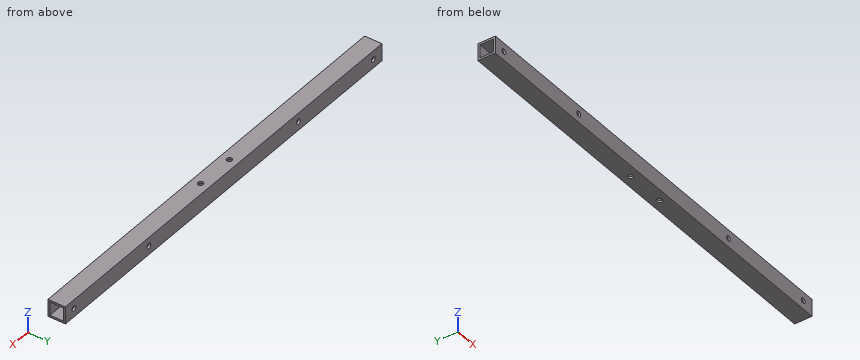
from build123d import *

# Parameters (mm, degrees)
SKETCH1_W           = 650
SKETCH1_H           = 26
BOSS_EXTRUDE1_DEPTH = 26
SHELL1_T            = -3
SKETCH2_R           = 4
CUT_EXTRUDE1_DEPTH  = 26
SKETCH3_R           = 4
CUT_EXTRUDE2_DEPTH  = 27


with BuildPart() as part:
    # Sketch1 → Boss-Extrude1 (new body)
    with BuildSketch(Plane(origin=(0, 0, 0), x_dir=(1, 0, 0), z_dir=(0, 1, 0))):
        Rectangle(SKETCH1_W, SKETCH1_H)
    extrude(amount=BOSS_EXTRUDE1_DEPTH)

    # Shell1
    shell1_openings = [part.faces().sort_by_distance(p)[0] for p in [
        (-325, 13, 0),
        (325, 13, 0),
    ]]
    offset(amount=SHELL1_T, openings=shell1_openings, kind=Kind.INTERSECTION)

    # Sketch2 → Cut-Extrude1 (cut)
    with BuildSketch(Plane(origin=(0, 26, 0), x_dir=(1, 0, 0), z_dir=(0, 1, 0))):
        with Locations((307.5, 0)):
            Circle(SKETCH2_R)
        with Locations((-307.5, 0)):
            Circle(SKETCH2_R)
        with Locations((153.75, 0)):
            Circle(SKETCH2_R)
        with Locations((-153.75, 0)):
            Circle(SKETCH2_R)
    extrude(amount=-CUT_EXTRUDE1_DEPTH, mode=Mode.SUBTRACT)

    # Sketch3 → Cut-Extrude2 (cut, through all)
    with BuildSketch(Plane.XY.offset(13)):
        with Locations((-29.5, 13)):
            Circle(SKETCH3_R)
        with Locations((29.5, 13)):
            Circle(SKETCH3_R)
    extrude(amount=-CUT_EXTRUDE2_DEPTH, mode=Mode.SUBTRACT)


solid = part.part
Geometry check sheet. Reference: the model listing, model coordinates, mm. Round coordinates to 2 decimals unless told otherwise and drop trailing zeros. Order: outer loops, then holes, each group sorted by start corner. A loop starts at its lowest first (then second) coordinate and runs counter-clockwise, first axis right, second up. Notation, with made-up numbers: M -27,41.5 L 18,41.5 A14 cw 18,53.5 Z; hole C -33,64 d8. An arc over 180 degrees is marked long. Write each question's results on one line, items separated by ' | '. Start each with the question number.
1. Material ranges on L1, parallel to X at y = 1.4, z = 0; L2, parallel to Y at x = 273.5, z = -7.5; L3, parallel to Z at x = -160.5, y = 10.25, recorded low to high. Write a range as from..to.
2. Go/stop test with flat-tipped pins: P1, Ø13, axis at x = -153.75, z = 0, coming from the -Y side; P2, Ø6.5, axis at x = -153.75, z = 0, coming from the +Y side. Record where each tip stops, or that it passes through.
3. Cross-section at C-C on z = 0. Give the number of separate pieces and of enclosed holes in the cut face, plus the area to 3 significant figures.
4. Cross-section at B-B on y = 13. Record the boundary of the cut face in (x, z), plus the area to 3 significant figures.
5. Cross-section at A-A on x = 11. Record the boundary of the cut face in (y, z).
Resolved:
1) L1: -325..-311.5, -303.5..-157.75, -149.75..149.75, 157.75..303.5, 311.5..325 | L2: 0..3, 23..26 | L3: -13..-10, 10..13
2) P1: y = 0 | P2: through
3) separate pieces: 10 | enclosed holes: 0 | area: 3,710 mm2
4) outline: M -325,-13 L -33.5,-13 L -33.5,-10 L -325,-10 Z; M -325,10 L -33.5,10 L -33.5,13 L -325,13 Z; M -25.5,-13 L 25.5,-13 L 25.5,-10 L -25.5,-10 Z; M -25.5,10 L 25.5,10 L 25.5,13 L -25.5,13 Z; M 33.5,-13 L 325,-13 L 325,-10 L 33.5,-10 Z; M 33.5,10 L 325,10 L 325,13 L 33.5,13 Z | area: 3,800 mm2
5) outline: M 0,-13 L 26,-13 L 26,13 L 0,13 Z; hole M 3,-10 L 23,-10 L 23,10 L 3,10 Z
